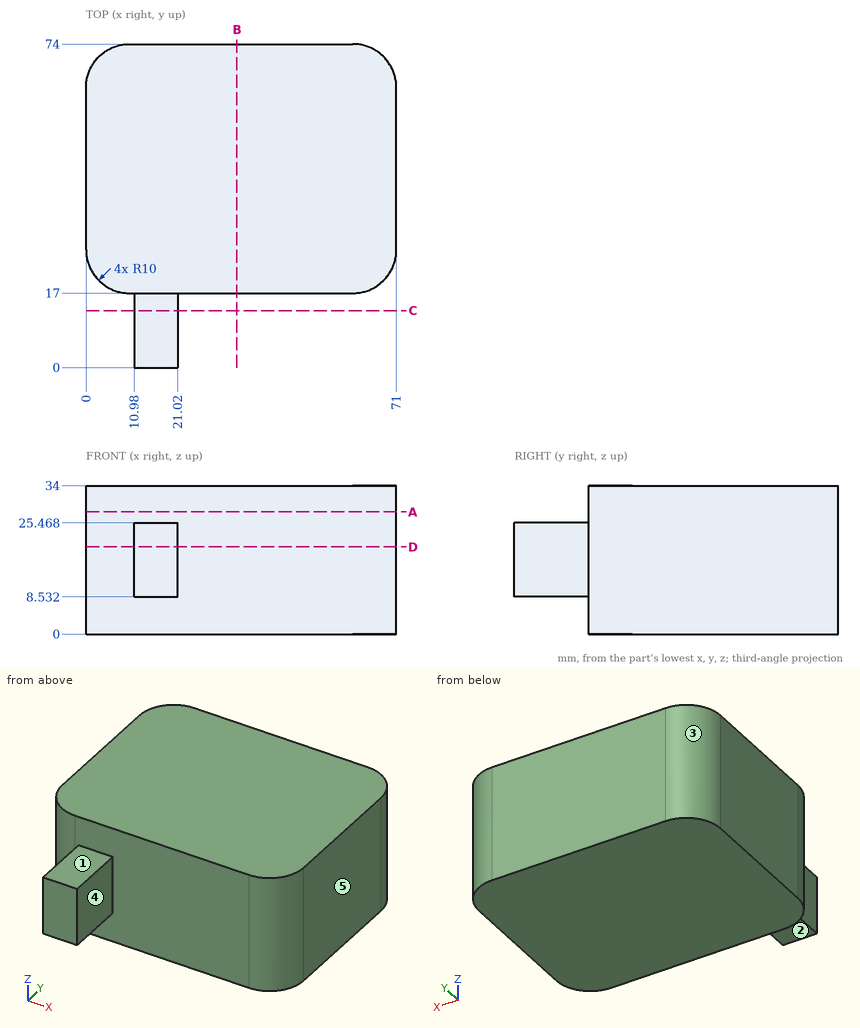
Design review of the part shown in the three views and the two pictorial views. Dimensions are in mm from the part's minimum x, y and z. A direction names the side the tool comes from. Round coordinates to 2 decimals unless told otherwise and drop trailing zeros. Write each loop counter-clockwise with the first axis right and the second up, starting at its lowest first coordinate (ties: lowest second). Pieces come first, ordered by that corner, then holes. Notation, with made-up numbers: (70.25, -13) -> (78.25, -13) arc R29 ccw to (78.25, 11) -> close; hole circle Ø11 at (-40, 78.25). An arc over 180 degrees is marked (long way). Write item = value, one per line. Start each with the question number.
1) Take a section at B-B, the plane x = 34.5. State the section outline as (y, z) points.
2) Take a section at D-D, the plane z = 20. State the section outline as (x, y) points.
3) Take a section at A-A, the plane z = 28. State the section outline as (x, y) points, plus the area to 3 significant figures.
4) Wall thickness on probe 1 along Y at (x, z) = (51.5, 23.5); probe 2 along X at (y, z) = (9, 21); probe 3 along Z at (x, y) = (20.5, 11): over which ranges is each line inside the solid? List them lowest first. Write a range as from..to.
5) Tool access review of the marked faces 1, 2, 3, 4 and 5: name each direction out of +Z, -Z, +X, -X, +Y, -Y from which nothing blocks a thin tool from reaching the whole face with its end or side.
6) Take a section at C-C, the plane y = 13. State the section outline as (x, z) points.
7) Clearance check with flat-ended pins moving along their axes: pin 1 (13.5 mm diameter, centred on y = 12.5, z = 20, fed in from -X); pin 2 (5 mm diameter, centred on x = 18.5, y = 4.5, fed in from -Z); pin 3 (12 mm diameter, centred on y = 19.5, z = 4, fed in from -X). State where each tip first meets the part, or that it passes through.
Results list:
q1.outline = (17, 0) -> (74, 0) -> (74, 34) -> (17, 34) -> close
q2.outline = (0, 27) arc R10 ccw to (10, 17) -> (10.98, 17) -> (10.98, 0) -> (21.02, 0) -> (21.02, 17) -> (61, 17) arc R10 ccw to (71, 27) -> (71, 64) arc R10 ccw to (61, 74) -> (10, 74) arc R10 ccw to (0, 64) -> close
q3.outline = (0, 27) arc R10 ccw to (10, 17) -> (61, 17) arc R10 ccw to (71, 27) -> (71, 64) arc R10 ccw to (61, 74) -> (10, 74) arc R10 ccw to (0, 64) -> close
q3.area = 3,960 mm²
q4.probe_1 = 17..74
q4.probe_2 = 10.98..21.02
q4.probe_3 = 8.53..25.47
q5.face_1 = +Z, +X, -X, -Y
q5.face_2 = -Z, +X, -X, -Y
q5.face_3 = +Z, -Z, -X, +Y
q5.face_4 = +Z, -Z, +X, -Y
q5.face_5 = +Z, -Z, +X, +Y, -Y
q6.outline = (10.98, 8.53) -> (21.02, 8.53) -> (21.02, 25.47) -> (10.98, 25.47) -> close
q7.pin_1 = 3.68
q7.pin_2 = 8.53
q7.pin_3 = 0.11
